The listing builds one solid part. Answer for the finished solid, in the listing's coordinates (mm). A direction names the side the tool comes from. Give positions to 0.01 mm unless a question says otherwise; leave off trailing zeros. Loops run counter-clockwise (first coordinate to the right, second up) from the corner with the lowest first, then second, coordinate; pieces in that order, holes last. Notation, with made-up numbers: M 45.5,30.5 L 98.5,30.5 A22 ccw 98.5,39.5 Z; hole C -35.5,-26.5 d8. An arc over 180 degrees is marked long. Use one line per item in the form item = value. Start each with the question number.
1. Each of these flat-tipped pins is pushed along its axis until it touches: pin 1 Ø9 at (x, y) = (68.5, -33) entering from +Z; pin 2 Ø2 at (x, z) = (43, 8.5) entering from -Y; pin 3 Ø1 at (y, z) = (-64.5, 19.5) entering from +X. Where does it stop, or does it pass through?
2. The part is cut by section A-A (x = 27). Write down the section's boundary in (y, z) (3 decimals), and give its area (3 significant figures).
3. The part is cut by section B-B (z = 3.5). Write down the section's boundary in (x, y), and give its area (3 significant figures).
4. For faces 4 (the face through (28, -84, 29.64)), 5 (the face through (51.603, -81.536, 28.778)), 6 (the face through (68, -20, 16.154)), determine the directions among +Z, -Z, +X, -X, +Y, -Y from which every point of the face is accessible in a straight line to the end or side of a thin tool.
5. The part is cut by section C-C (z = 23). Give the number of separate pieces and of enclosed holes in the cut face, and give its area (3 significant figures).
6. Straight lines are drawn through the part: line 1 (Z direction, x = 65, y = -59.5); line 2 (Y direction, x = 68.5, z = 13); line 3 (X direction, y = -2, z = 19.5). For each, find the intervals that lie inside material, in ascending order. Write a range as from..to.
7. The mould has two halves that part along Z. Classify faces 1 (the face through (60, 4, 29.64)), 2 (the face through (-4, -47, 24.13)), 3 (the face through (31, -79.616, 20)): released by +Z, released by -Z, zero draft, split by the parting line, or undercut.
8. The part is cut by section D-D (x = 19). Write down the section's boundary in (y, z) (3 decimals).
from build123d import *

# Parameters (mm, degrees)
F0_W      = 80
F0_H      = 96
F0_W_2    = 63.8302
F0_H_2    = 79.6163
F1_DEPTH  = 27.94
F2_W      = 80
F2_H      = 96
F2_W_2    = 63.8302
F2_H_2    = 79.6163
F3_DEPTH  = 2.54
F4_W      = 63.8302
F4_H      = 79.6163
F5_DEPTH  = 8.255
F6_W      = 7.62
F6_H      = 8.89
F7_DEPTH  = 25.4
F9_DEPTH  = 19.05
F10_W     = 11.9634
F10_H     = 6.35
F11_DEPTH = 127
F12_R     = 2.4
F13_DEPTH = 1.7


# Not quite as in the source:
# - a feature names something its author has since deleted; it is built from what else it names


with BuildPart() as f1:
    # F0 (on Top) → F1 (new body)
    with BuildSketch(Plane.XY):
        with Locations((31.9151, -39.9151)):
            Rectangle(F0_W, F0_H)
        with Locations((31.9151, -39.80815)):
            Rectangle(F0_W_2, F0_H_2, mode=Mode.SUBTRACT)
    extrude(amount=F1_DEPTH)

    # F2 (on Top) → F3 (join)
    with BuildSketch(Plane.XY):
        with Locations((31.9151, -39.9151)):
            Rectangle(F2_W, F2_H)
        with Locations((31.9151, -39.80815)):
            Rectangle(F2_W_2, F2_H_2, mode=Mode.SUBTRACT)
        with Locations((31.9151, -39.80815)):
            Rectangle(F2_W_2, F2_H_2)
    extrude(amount=-F3_DEPTH)

    # F4 (on face) → F5 (join)
    with BuildSketch(Plane.XY):
        with Locations((31.9151, -39.80815)):
            Rectangle(F4_W, F4_H)
        with BuildLine():
            ThreePointArc((14.01445, -15.14475), (16.6182707153, -8.8585707153), (22.90445, -6.25475))
            Line((22.90445, -6.25475), (40.93845, -6.25475))
            ThreePointArc((40.93845, -6.25475), (47.2246292847, -8.8585707153), (49.82845, -15.14475))
            Line((49.82845, -15.14475), (49.82845, -63.40475))
            ThreePointArc((49.82845, -63.40475), (47.2246292847, -69.6909292847), (40.93845, -72.29475))
            Line((40.93845, -72.29475), (35.73145, -72.29475))
            Line((35.73145, -72.29475), (35.73145, -73.81875))
            Line((35.73145, -73.81875), (32.30245, -73.81875))
            Line((32.30245, -73.81875), (31.92145, -73.81875))
            Line((31.92145, -73.81875), (28.11145, -73.81875))
            Line((28.11145, -73.81875), (28.11145, -72.29475))
            Line((28.11145, -72.29475), (22.90445, -72.29475))
            ThreePointArc((22.90445, -72.29475), (16.6182707153, -69.6909292847), (14.01445, -63.40475))
            Line((14.01445, -63.40475), (14.01445, -15.14475))
        make_face(mode=Mode.SUBTRACT)
    extrude(amount=F5_DEPTH)

    # F6 (on face) → F7 (cut)
    with BuildSketch(Plane.XZ.offset(87.9151)):
        Polygon((39.5351, 8.89), (31.9151, 8.89), (31.9151, 0), (36.9951, 0), (39.5351, 0), align=None)
        with Locations((28.1051, 4.445)):
            Rectangle(F6_W, F6_H)
    extrude(amount=-F7_DEPTH, mode=Mode.SUBTRACT)

    # F8 (on face) → F9 (cut)
    with BuildSketch(Plane.XZ.offset(87.9151)):
        Polygon((28.1432, 13.589), (16.1798, 13.589), (16.1798, 7.239), (24.2951, 7.239), (24.2951, 8.89), (28.1432, 8.89), align=None)
        Polygon((35.687, 13.589), (35.687, 8.89), (39.5351, 8.89), (39.5351, 7.239), (47.6504, 7.239), (47.6504, 13.589), align=None)
    extrude(amount=-F9_DEPTH, mode=Mode.SUBTRACT)

    # F10 (on face) → F11 (cut)
    with BuildSketch(Plane.YZ.offset(71.9151)):
        with Locations((-33.2984, 20.955)):
            Rectangle(F10_W, F10_H)
        with Locations((-20.065, 20.955)):
            Rectangle(F10_W, F10_H)
        with Locations((-46.5318, 20.955)):
            Rectangle(F10_W, F10_H)
        with Locations((-59.7652, 20.955)):
            Rectangle(F10_W, F10_H)
        with Locations((-20.065, 12.9794)):
            Rectangle(F10_W, F10_H)
        with Locations((-33.2984, 12.9794)):
            Rectangle(F10_W, F10_H)
        with Locations((-46.5318, 12.9794)):
            Rectangle(F10_W, F10_H)
        with Locations((-59.7652, 12.9794)):
            Rectangle(F10_W, F10_H)
    extrude(amount=-F11_DEPTH, mode=Mode.SUBTRACT)

    # F12 (on face) → F13 (join)
    with BuildSketch(Plane.XY.offset(27.94)):
        with Locations((-4.0849, -83.9151)):
            Circle(F12_R)
        with Locations((3.9151, -83.9151)):
            Circle(F12_R)
        with Locations((11.9151, -83.9151)):
            Circle(F12_R)
        with Locations((19.9151, -83.9151)):
            Circle(F12_R)
        with Locations((27.9151, -83.9151)):
            Circle(F12_R)
        with Locations((35.9151, -83.9151)):
            Circle(F12_R)
        with Locations((43.9151, -83.9151)):
            Circle(F12_R)
        with Locations((51.9151, -83.9151)):
            Circle(F12_R)
        with Locations((67.9151, -83.9151)):
            Circle(F12_R)
        with Locations((59.9151, -83.9151)):
            Circle(F12_R)
        with Locations((67.9151, -75.9151)):
            Circle(F12_R)
        with Locations((67.9151, -67.9151)):
            Circle(F12_R)
        with Locations((67.9151, -59.9151)):
            Circle(F12_R)
        with Locations((67.9151, -51.9151)):
            Circle(F12_R)
        with Locations((67.9151, -43.9151)):
            Circle(F12_R)
        with Locations((67.9151, -35.9151)):
            Circle(F12_R)
        with Locations((67.9151, -27.9151)):
            Circle(F12_R)
        with Locations((67.9151, -19.9151)):
            Circle(F12_R)
        with Locations((67.9151, -11.9151)):
            Circle(F12_R)
        with Locations((67.9151, -3.9151)):
            Circle(F12_R)
        with Locations((-4.0849, -75.9151)):
            Circle(F12_R)
        with Locations((-4.0849, -67.9151)):
            Circle(F12_R)
        with Locations((-4.0849, -59.9151)):
            Circle(F12_R)
        with Locations((-4.0849, -51.9151)):
            Circle(F12_R)
        with Locations((-4.0849, -43.9151)):
            Circle(F12_R)
        with Locations((-4.0849, -35.9151)):
            Circle(F12_R)
        with Locations((-4.0849, -27.9151)):
            Circle(F12_R)
        with Locations((-4.0849, -19.9151)):
            Circle(F12_R)
        with Locations((-4.0849, -11.9151)):
            Circle(F12_R)
        with Locations((-4.0849, -3.9151)):
            Circle(F12_R)
        with Locations((-4.0849, 4.0849)):
            Circle(F12_R)
        with Locations((3.9151, 4.0849)):
            Circle(F12_R)
        with Locations((11.9151, 4.0849)):
            Circle(F12_R)
        with Locations((19.9151, 4.0849)):
            Circle(F12_R)
        with Locations((27.9151, 4.0849)):
            Circle(F12_R)
        with Locations((59.9151, 4.0849)):
            Circle(F12_R)
        with Locations((51.9151, 4.0849)):
            Circle(F12_R)
        with Locations((43.9151, 4.0849)):
            Circle(F12_R)
        with Locations((35.9151, 4.0849)):
            Circle(F12_R)
        with Locations((67.9151, 4.0849)):
            Circle(F12_R)
    extrude(amount=F13_DEPTH)


solid = f1.part
Derived:
q1.pin_1 = 29.64
q1.pin_2 = -6.79
q1.pin_3 = through
q2.outline = M -87.915,-2.54 L 8.085,-2.54 L 8.085,27.94 L 6.304,27.94 L 6.304,29.64 L 1.866,29.64 L 1.866,27.94 L 0,27.94 L 0,8.255 L -6.255,8.255 L -6.255,0 L -87.915,0 Z; M -87.915,13.589 L -79.616,13.589 L -79.616,27.94 L -81.696,27.94 L -81.696,29.64 L -86.134,29.64 L -86.134,27.94 L -87.915,27.94 Z
q2.area = 656 mm2
q3.outline = M -8.08,-87.92 L 24.3,-87.92 L 24.3,-72.29 L 22.9,-72.29 A8.89 cw 14.01,-63.4 L 14.01,-15.14 A8.89 cw 22.9,-6.25 L 40.94,-6.25 A8.89 cw 49.83,-15.14 L 49.83,-63.4 A8.89 cw 40.94,-72.29 L 39.54,-72.29 L 39.54,-87.92 L 71.92,-87.92 L 71.92,8.08 L -8.08,8.08 Z
q3.area = 5,140 mm2
q4.face_4 = +Z, +X, -X, +Y, -Y
q4.face_5 = +Z
q4.face_6 = +X, -X
q5.separate_pieces = 8
q5.enclosed_holes = 0
q5.area = 1,820 mm2
q6.line_1 = -2.54..9.8, 16.15..17.78, 24.13..27.94
q6.line_2 = -87.92..-65.75, -53.78..-52.51, -40.55..-39.28, -27.32..-26.05, -14.08..8.08
q6.line_3 = -8.08..0, 63.83..71.92
q7.face_1 = released by +Z
q7.face_2 = undercut
q7.face_3 = zero draft
q8.outline = M -87.915,-2.54 L 8.085,-2.54 L 8.085,27.94 L 6.304,27.94 L 6.304,29.64 L 1.866,29.64 L 1.866,27.94 L 0,27.94 L 0,8.255 L -7.158,8.255 L -7.158,0 L -71.391,0 L -71.391,7.239 L -87.915,7.239 Z; M -87.915,13.589 L -79.616,13.589 L -79.616,27.94 L -81.696,27.94 L -81.696,29.64 L -86.134,29.64 L -86.134,27.94 L -87.915,27.94 Z
